Can you work these out from the model? Positions are in its coordinate system, mm. A direction names the side the tool comes from. Round coordinates to 2 decimals unless told otherwise and drop trailing zeros. Order: outer loops, then holes, each group sorted by start corner. A loop starts at its lowest first (then second) coordinate and runs counter-clockwise, first axis right, second up. Notation, with made-up numbers: (79, 73.5) - (102, 73.5) arc R14 cw to (102, 98.5) - close; hole circle Ø11 at (77.5, 11). An arc over 180 degrees is marked (long way). Write item = value, one per line.
Autodesk Inventor part; units mm, degrees
ref_plane "YZ Plane" through (0, 0, 0) normal (1, 0, 0) x (0, 1, 0)
ref_plane "XZ Plane" through (0, 0, 0) normal (0, 1, 0) x (-1, 0, 0)
ref_plane "XY Plane" through (0, 0, 0) normal (0, 0, 1) x (1, 0, 0)
sketch "Skizze1" plane through (0, 0, 0) normal (1, 0, 0) x (0, 1, 0)
  circle A0 centre (0, 0) radius 17.5
  dimension "d0" = 35
extrude "Extrusion1" add sketch "Skizze1" along normal blind 35
sketch "Skizze2" plane through (35, 0, 0) normal (1, 0, 0) x (0, 0, -1)
  circle A0 centre (0, 0) radius 4.5
  dimension "d3" = 9
extrude "Extrusion2" add sketch "Skizze2" along normal blind 2
sketch "Skizze3" plane through (37, 0, 0) normal (1, 0, 0) x (0, 0, -1)
  circle A0 centre (0, 0) radius 4.5
  circle A1 centre (0, 0) radius 4
  dimension "d6" = 8
extrude "Extrusion3" add sketch "Skizze3" along normal blind 14 contours A1
thread "Gewinde1"
properties part number "Spannrolle Durchmesser 30mm Breite 35mm"
(1) Will these pins go through, and if not, where does the flat tip stop? P1, Ø6, axis at x = 29, y = -4.5, coming from the -Z side; P2, Ø4, axis at x = 25.5, z = 8, coming from the -Y side; P3, Ø6, axis at x = 16, z = 7.5, coming from the +Y side.
Computed:
P1 = -17.44
P2 = -16.44
P3 = 16.91
(2) If we section it at A-A (z = 0): Write out the boundary of the cut face in (x, y).
Computed:
outline = (0, -17.5) - (35, -17.5) - (35, -4.5) - (37, -4.5) - (37, -4) - (51, -4) - (51, 4) - (37, 4) - (37, 4.5) - (35, 4.5) - (35, 17.5) - (0, 17.5) - close
(3) If we section it at D-D (x = 29): Write out the boundary of the cut face in (y, z).
Computed:
outline = circle Ø35 at (0, 0)
(4) On a 3-axis mill with a long thin cutter (end or side, diameter ignored), from which of +Z, -Z, +X, -X, +Y, -Y can I reach the whole of each face in a straight line? I mean faces 1 (the face through (35.99, -4.46, 0.59)), 2 (the face through (51, 0, 0)). Say none if no direction works.
Computed:
face_1 = +X
face_2 = +Z, -Z, +X, +Y, -Y
(5) If we section it at C-C (x = 39.5): Write out the boundary of the cut face in (y, z), plus the area to 3 significant figures.
Computed:
outline = circle Ø8 at (0, 0)
area = 50.3 mm^2
(6) If I drill on line 1 (X direction, y = -10, z = -7); line 2 (Y direction, x = 31, z = -0.5); line 3 (Y direction, x = 34, z = 5), over which ranges is the centre line in solid material (lowest first)? Write a range as from..to.
Computed:
line_1 = 0..35
line_2 = -17.49..17.49
line_3 = -16.77..16.77
